```python
from build123d import *

# Parameters (mm, degrees)
F1_DEPTH = 63.5
F0_W     = 27.6548634248
F0_H     = 19.05
F0_H_2   = 4.7498
F0_H_3   = 4.7752
F2_DEPTH = 25.4
F3_DEPTH = 19.05
F4_R     = 6.35
F5_R     = 6.35


with BuildPart() as f1:
    # F0 (on Front) → F1 (new body, symmetric)
    with BuildSketch(Plane.XZ):
        Polygon((-41.275, -9.525), (41.275, -9.525), (41.275, 9.525), (22.225, 9.525), (-41.275, 9.525), align=None)
    extrude(amount=F1_DEPTH, both=True)

    # F0 (on Front) → F2 (join, symmetric)
    with BuildSketch(Plane.XZ):
        with BuildLine():
            Line((22.225, 9.525), (41.275, 9.525))
            Line((41.275, 9.525), (41.275, 27.0002))
            ThreePointArc((41.275, 27.0002), (45.9246798487, 38.2255201513), (57.15, 42.8752))
            Line((57.15, 42.8752), (58.0701365752, 42.8752))
            Line((58.0701365752, 42.8752), (58.0701365752, 61.9252))
            Line((58.0701365752, 61.9252), (57.15, 61.9252))
            ThreePointArc((57.15, 61.9252), (32.4542956671, 51.6959043329), (22.225, 27.0002))
            Line((22.225, 27.0002), (22.225, 9.525))
        make_face()
        with Locations((71.8975682876, 52.4002)):
            Rectangle(F0_W, F0_H)
        Polygon((85.725, 66.675), (85.725, 61.9252), (85.725, 42.8752), (85.725, 38.1), (108.8701365752, 38.1), (108.8701365752, 66.675), align=None)
        with Locations((71.8975682876, 64.3001)):
            Rectangle(F0_W, F0_H_2)
        with Locations((71.8975682876, 40.4876)):
            Rectangle(F0_W, F0_H_3)
    extrude(amount=F2_DEPTH, both=True)

    # F0 (on Front) → F3 (join)
    with BuildSketch(Plane.XZ):
        with BuildLine():
            add(Edge.make_bspline(
                [(-41.275, 9.525), (-41.7954027653, 31.1398338526), (19.2923080176, 62.1306672692), (57.15, 61.9252)],
                knots=[0, 0, 0, 0, 111.5045361635, 111.5045361635, 111.5045361635, 111.5045361635], degree=3))
            Line((-41.275, 9.525), (22.225, 9.525))
            Line((22.225, 9.525), (22.225, 27.0002))
            ThreePointArc((22.225, 27.0002), (32.4542956671, 51.6959043329), (57.15, 61.9252))
        make_face()
    extrude(amount=F3_DEPTH)

    # F4
    f4_edges = [f1.edges().sort_by_distance(p)[0] for p in [
        (41.275, -63.5, 0),
        (-41.275, -63.5, 0),
    ]]
    fillet(f4_edges, radius=F4_R)

    # F5
    f5_edges = [f1.edges().sort_by_distance(p)[0] for p in [
        (41.275, 63.5, 0),
        (-41.275, 63.5, 0),
    ]]
    fillet(f5_edges, radius=F5_R)


solid = f1.part
```
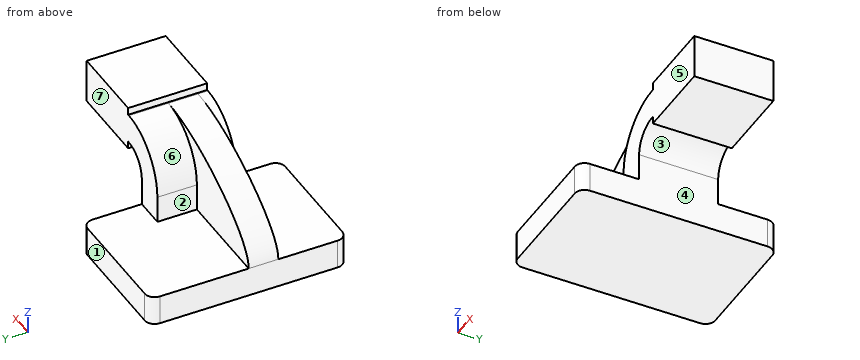
Geometry check sheet. Reference: the model listing, model coordinates, mm. Face numbers are marked on the shaded views. A direction names the side the tool comes from. Coordinates: 2 decimals unless noted, no trailing zeros. Order: outer loops, then holes, each group sorted by start corner. A loop starts at its lowest first (then second) coordinate and runs counter-clockwise, first axis right, second up.
Item 1: Depth check by flat-ended pin: pin 1 (1 mm diameter, centred on x = 58, y = -8.5, fed in from -Z); pin 2 (8 mm diameter, centred on x = 21, z = 48.5, fed in from +Y); pin 3 (2.5 mm diameter, centred on y = -5.5, z = 64.5, fed in from -X). Enter the tip coordinate at first touch or a pass-through.
Item 2: Tool access check on the marked faces 5, 6 and 7. Record the directions out of +Z, -Z, +X, -X, +Y, -Y that give a thin tool (end or side, any length) a straight path to the whole face; none if there is none.
Item 3: Scan lines: line 1 along X through (y, z) = (41, -2) (3 decimals); line 2 along Y through (x, z) = (102, 47.5); line 3 along Y through (x, z) = (11, 45.5). Record each from-to range of solid material in increasing order.
Item 4: Section check A-A (y = 29). Enter the section's corners in (x, z) (3 decimals), plus the area to 3 significant figures.
Item 5: Mould release check, pull along X, two halves, no side actions. Record for the marked faces 1, 2, 3 and 4: released by +X, released by -X, zero draft, split by the parting line, or undercut.
Check sheet entries:
1. pin 1: stops at z = 38.1
1. pin 2: stops at y = 0
1. pin 3: stops at x = 58.07
2. face 5: +Z, +X, -X, -Y
2. face 6: +Z, -X, +Y
2. face 7: +Z, +X, -X, +Y
3. line 1: x = -41.275 to 41.275
3. line 2: y = -25.4 to 25.4
3. line 3: y = -19.05 to 0
4. outline: (-41.275, -9.525) - (41.275, -9.525) - (41.275, 9.525) - (-41.275, 9.525) - close
4. area: 1,570 mm2
5. face 1: zero draft
5. face 2: released by -X
5. face 3: undercut
5. face 4: released by +X
